Verification items for this drawing (mm, ordinates from the low corner). Coordinates: 2 decimals unless noted, no trailing zeros. Order: outer loops, then holes, each group sorted by start corner. A loop starts at its lowest first (then second) coordinate and runs counter-clockwise, first axis right, second up. Notation, with made-up numbers: (3, 42) - (58, 42) arc R18 ccw to (58, 76) - close; hole circle Ø6 at (-10.5, -32.75). An arc over 180 degrees is marked (long way). Use CSV: the item, a comma, the result in double quotes. Start each with the question number.
1) Depth check by flat-ended pin: P1, Ø1.5, axis at y = 44.45, z = 7.94, coming from the -X side; P2, Ø4, axis at y = 49.2, z = 7.94, coming from the +X side. Enter the tip coordinate at first touch or a pass-through.
2) Thickness scan on probe 1 along Z at (x, y) = (1.25, 30.2) (1 decimal); probe 2 along Y at (x, z) = (1.2, 11) (1 decimal); probe 3 along Y at (x, z) = (1, 4.75) (1 decimal). Record the ranges inside material, lowest first. Write a range as [from, to].
3) Sectioned sample at C-C, the plane z = 10. Record the cut outline in (x, y), and give its area (3 significant figures).
4) Sectioned sample at B-B, the plane x = 0.8. Count the separate pieces of the cut face and the enclosed holes in it, and give its area (4 significant figures).
5) Sectioned sample at A-A, the plane y = 53.95. Record the cut outline in (x, z) (1 decimal).
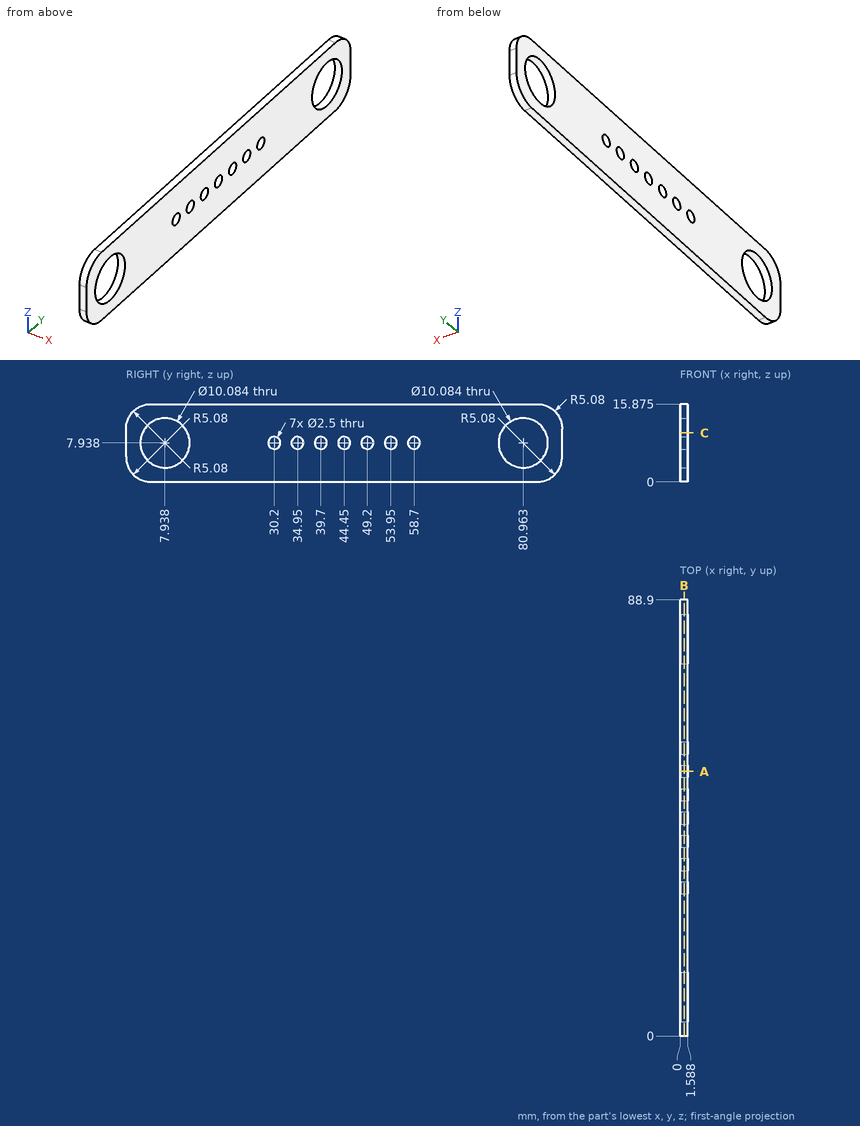
Evaluation:
1,P1,"through"
1,P2,"x = 1.59"
2,probe 1,"[0, 6.7], [9.2, 15.9]"
2,probe 2,"[0, 3.9], [11.9, 77], [85, 88.9]"
2,probe 3,"[0, 4], [11.8, 77.1], [84.9, 88.9]"
3,outline,"(0, 0) - (1.59, 0) - (1.59, 3.34) - (0, 3.34) - close; (0, 12.54) - (1.59, 12.54) - (1.59, 76.36) - (0, 76.36) - close; (0, 85.56) - (1.59, 85.56) - (1.59, 88.9) - (0, 88.9) - close"
3,area,"112 mm²"
4,separate pieces,"1"
4,enclosed holes,"9"
4,area,"1,195 mm²"
5,outline,"(0, 0) - (1.6, 0) - (1.6, 6.7) - (0, 6.7) - close; (0, 9.2) - (1.6, 9.2) - (1.6, 15.9) - (0, 15.9) - close"
